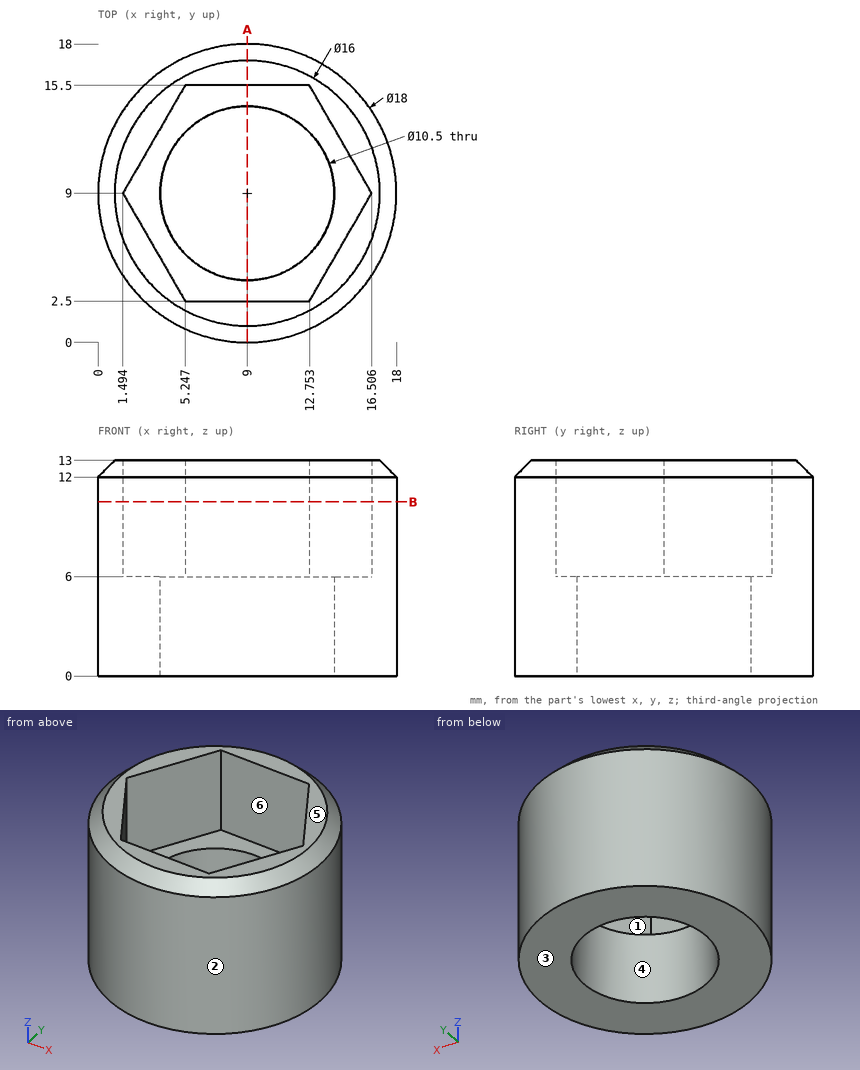
For this review, use the dimensioned drawing (mm, ordinates from the lowest corner) and the shaded views. A direction names the side the tool comes from. Round coordinates to 2 decimals unless told otherwise and drop trailing zeros. Order: outer loops, then holes, each group sorted by start corner. A loop starts at its lowest first (then second) coordinate and runs counter-clockwise, first axis right, second up. Notation, with made-up numbers: (84.5, 53) -> (130.5, 53) arc R30 cw to (130.5, 77) -> close; hole circle Ø10 at (35, -39.75). An arc over 180 degrees is marked (long way). Write item = value, one per line. Start each with the question number.
Item 1: Consider section B-B on z = 10.5. Write out the cut boundary in (x, y) (1 decimal).
Item 2: Mouldability with a two-part tool opening along X and no side actions: class the marked faces 1, 2, 3 and 4 as released by +X, released by -X, zero draft, split by the parting line, or undercut.
Item 3: Consider section A-A on x = 9. Write out the cut boundary in (y, z).
Item 4: For the marked faces 5 and 6, list the 3-axis set-ups (+Z, -Z, +X, -X, +Y, -Y) from which the entire face can be reached by the end or side of a thin tool; tool diameter is ignored.
Item 5: For line 1 along Y through (x, z) = (9, 3.05); line 2 along X through (y, z) = (9.5, 4.75); line 3 along Z through (x, y) = (5.75, 13.5), list the stretches that pass through material, from the lowest coordinate up.
Item 6: Clearance check with flat-ended pins moving along their axes: pin 1 Ø6 at (x, z) = (15, 2.5) entering from -Y (1 decimal); pin 2 Ø1 at (x, y) = (10, 14) entering from +Z; pin 3 Ø6 at (y, z) = (4, 2.5) entering from -X (1 decimal); pin 4 Ø3 at (x, y) = (2, 9.5) entering from -Z. State where each tip first meets the part, or that it passes through.
Conclusion:
q1.outline = circle Ø18 at (9, 9); hole (1.5, 9) -> (5.2, 2.5) -> (12.8, 2.5) -> (16.5, 9) -> (12.8, 15.5) -> (5.2, 15.5) -> close
q2.face_1 = undercut
q2.face_2 = split by the parting line
q2.face_3 = zero draft
q2.face_4 = undercut
q3.outline = (0, 0) -> (3.75, 0) -> (3.75, 6) -> (2.5, 6) -> (2.5, 13) -> (1, 13) -> (0, 12) -> close; (14.25, 0) -> (18, 0) -> (18, 12) -> (17, 13) -> (15.5, 13) -> (15.5, 6) -> (14.25, 6) -> close
q4.face_5 = +Z, +X, -X, +Y, -Y
q4.face_6 = +Z
q5.line_1 = 0 to 3.75, 14.25 to 18
q5.line_2 = 0.01 to 3.77, 14.23 to 17.99
q5.line_3 = 0 to 6
q6.pin_1 = 0.5
q6.pin_2 = 6
q6.pin_3 = 0.2
q6.pin_4 = 0
